Work out the finished part from the listing and answer in its coordinate system (mm). Face numbers are marked on the shaded views. A direction names the side the tool comes from. Give positions to 0.01 mm unless a question says otherwise; leave off trailing zeros. Loops run counter-clockwise (first coordinate to the right, second up) from the corner with the lowest first, then second, coordinate; pieces in that order, holes last.
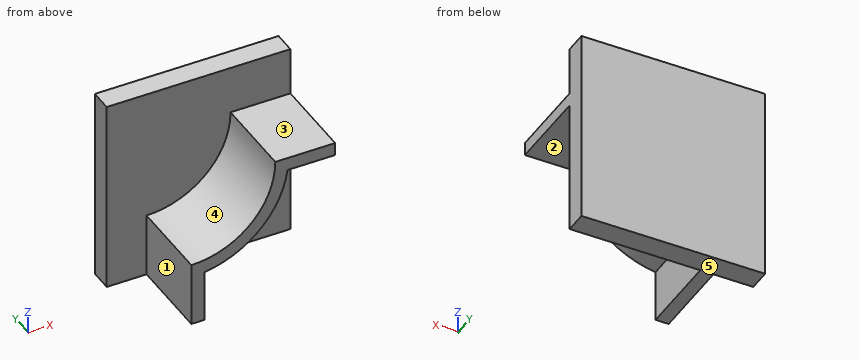
from build123d import *

# Parameters (mm, degrees)
F0_W     = 210
F0_H     = 225
F1_DEPTH = 25.4
F4_DEPTH = 96


with BuildPart() as f1:
    # F0 (on Front) → F1 (new body)
    with BuildSketch(Plane.XZ):
        with Locations((-25.301798, 8.873123)):
            Rectangle(F0_W, F0_H)
    extrude(amount=F1_DEPTH)


with BuildPart() as f1_1:
    # F2: moved
    add(f1.part.moved(Location((25.4, 0, -8.763))))

    # F3 (on face) → F4 (join)
    with BuildSketch(Plane.XZ.offset(25.4)):
        with BuildLine():
            Line((-59.321807, -38.761023), (-59.321807, -112.389877))
            Line((-59.321807, -112.389877), (-44.321807, -112.389877))
            Line((-44.321807, -112.389877), (-44.321807, -52.74284))
            ThreePointArc((-44.321807, -52.74284), (19.167046, -21.249876), (50.66001, 42.238977))
            Line((50.66001, 42.238977), (105.098202, 42.238977))
            Line((105.098202, 42.238977), (105.098202, 57.238977))
            Line((105.098202, 57.238977), (36.678193, 57.238977))
            ThreePointArc((36.678193, 57.238977), (8.560444, -10.643274), (-59.321807, -38.761023))
        make_face()
    extrude(amount=F4_DEPTH)


solid = f1_1.part
Item 1: Find section A-A, the plane y = -57.5. Write down the section's boundary in (x, z), plus the area to 3 significant figures.
Item 2: For the marked faces 1, 2, 3, 4 and 5, determine the directions among +Z, -Z, +X, -X, +Y, -Y from which every point of the face is accessible in a straight line to the end or side of a thin tool.
Item 3: Flat-ended cylindrical pins translate along their axes: pin 1 Ø2 at (x, y) = (-54, -39.5) entering from +Z; pin 2 Ø1 at (y, z) = (-67.5, -10) entering from -X; pin 3 Ø5 at (x, z) = (79.5, 60) entering from -Y. Find the tip coordinate at first contact, or state that the pin passes through.
Item 4: Find section B-B, the plane x = 84.5. Write down the section's boundary in (y, z), plus the area to 4 significant figures.
Item 5: Find section D-D, the plane x = -54.5. Write down the section's boundary in (y, z).
Item 6: Find section C-C, the plane z = 50. Write down the section's boundary in (x, y), plus the area to 3 significant figures.
Item 7: Consider line 1 (Y direction, x = -30.5, z = 89.5); line 2 (Z direction, x = 92, y = -61); line 3 (X direction, y = -91.5, z = 56). Determine where each line is inside the solid, lowest interval first.
Ans:
1. outline: (-59.32, -112.39) - (-44.32, -112.39) - (-44.32, -52.74) arc R111 ccw to (50.66, 42.24) - (105.1, 42.24) - (105.1, 57.24) - (36.68, 57.24) arc R96 cw to (-59.32, -38.76) - close
1. area: 4,130 mm2
2. face 1: +Z, -Z, -X, -Y
2. face 2: -Z, +X, -Y
2. face 3: +Z, +X, -X, -Y
2. face 4: +Z, -X, -Y
2. face 5: -Z, +X, -X, +Y, -Y
3. pin 1: stops at z = -38.55
3. pin 2: stops at x = 8.7
3. pin 3: stops at y = -25.4
4. outline: (-121.4, 42.24) - (-25.4, 42.24) - (-25.4, -112.39) - (0, -112.39) - (0, 112.61) - (-25.4, 112.61) - (-25.4, 57.24) - (-121.4, 57.24) - close
4. area: 7,155 mm2
5. outline: (-121.4, -112.39) - (0, -112.39) - (0, 112.61) - (-25.4, 112.61) - (-25.4, -38.64) - (-121.4, -38.64) - close
6. outline: (-104.9, -25.4) - (36.4, -25.4) - (36.4, -121.4) - (105.1, -121.4) - (105.1, 0) - (-104.9, 0) - close
6. area: 11,900 mm2
7. line 1: y = -25.4 to 0
7. line 2: z = 42.24 to 57.24
7. line 3: x = 36.67 to 105.1
